```python
from build123d import *

# Parameters (mm, degrees)
SKETCH1_W          = 2.5
SKETCH1_H          = 4.1
CUT_EXTRUDE1_DEPTH = 18.4


with BuildPart() as part:
    # Sketch1 → Revolve1 (revolve)
    with BuildSketch(Plane.XY, mode=Mode.PRIVATE) as revolve1_sk:
        with Locations((0, 7.15)):
            Rectangle(SKETCH1_W, SKETCH1_H)
    revolve(revolve1_sk.sketch.rotate(Axis((1.25, 0, 0), (-1, 0, 0)), 90), axis=Axis((1.25, 0, 0), (-1, 0, 0)))

    # Sketch2 → Cut-Extrude1 (cut)
    with BuildSketch(Plane.XY):
        Polygon((-1.427121141, 0.26622761), (-1.25, -0.738276298), (1.427121141, -0.26622761), (1.25, 0.738276298), align=None)
    extrude(amount=CUT_EXTRUDE1_DEPTH, mode=Mode.SUBTRACT)


solid = part.part
```
Verification items for the finished model (mm, model axes). A direction names the side the tool comes from. Give positions to 0.01 mm unless a question says otherwise; leave off trailing zeros. Write each loop counter-clockwise with the first axis right and the second up, starting at its lowest first coordinate (ties: lowest second). Pieces come first, ordered by that corner, then holes. Notation, with made-up numbers: M -27.5,14 L 12.5,14 A30 cw 12.5,50 Z; hole C 76.25,85 d1. An arc over 180 degrees is marked long. One line per question, with ' | ' between items.
1) Set-up check for faces 3 (the flat face through (-1.25, 4, 4)), 4 (the flat face through (-0.02, -0.52, 7.09)): record each of +Z, -Z, +X, -X, +Y, -Y from which the full face is reachable in a straight line by a thin tool's end or side.
Result:
face 3: +Z, -Z, -X, +Y, -Y | face 4: +Z, -X
2) Mould release check, pull along Y, two halves, no side actions. Record for faces 1 (the flat face through (1.25, 4, 4)), 2 (the flat face through (0.02, 0.52, 7.09)): released by +Y, released by -Y, zero draft, split by the parting line, or undercut.
Result:
face 1: zero draft | face 2: undercut
3) Section check A-A on z = 0. Enter the section's corners in (x, y), plus the area to 3 significant figures.
Result:
outline: M -1.25,-9.2 L 1.25,-9.2 L 1.25,-5.1 L -1.25,-5.1 Z; M -1.25,5.1 L 1.25,5.1 L 1.25,9.2 L -1.25,9.2 Z | area: 20.5 mm2
4) Section check C-C on x = -0.9. Enter the section's corners in (y, z).
Result:
outline: M -0.68,5.05 L -0.68,9.18 A9.2 ccw long 0.36,9.19 L 0.36,5.09 A5.1 cw long Z
5) Section check B-B on y = 1.25. Enter the section's corners in (x, z).
Result:
outline: M -1.25,-9.11 L 1.25,-9.11 L 1.25,-4.94 L -1.25,-4.94 Z; M -1.25,4.94 L 1.25,4.94 L 1.25,9.11 L -1.25,9.11 Z
6) Section check D-D on z = -6. Enter the section's corners in (x, y).
Result:
outline: M -1.25,-6.97 L 1.25,-6.97 L 1.25,6.97 L -1.25,6.97 Z
7) Thickness scan on line 1 along Z through (x, y) = (0.35, 3.25); line 2 along Y through (x, z) = (0.05, -3); line 3 along Z through (x, y) = (0.1, -1.5). Record the ranges inside material, lowest first. Write a range as [from, to].
Result:
line 1: z = [-8.61, -3.93], [3.93, 8.61] | line 2: y = [-8.7, -4.12], [4.12, 8.7] | line 3: z = [-9.08, -4.87], [4.87, 9.08]
